The model under review builds one solid part; all positions refer to its coordinate system, in mm. Face numbers are marked on the shaded views. A direction names the side the tool comes from. Coordinates: 2 decimals unless noted, no trailing zeros. Order: outer loops, then holes, each group sorted by start corner. A loop starts at its lowest first (then second) coordinate and runs counter-clockwise, first axis right, second up.
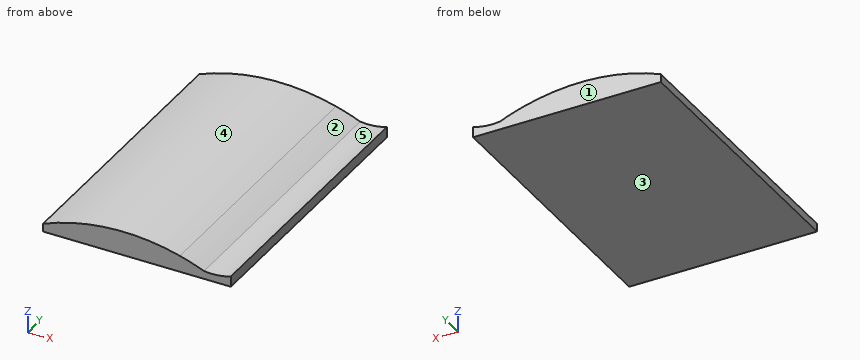
```python
from build123d import *

# Parameters (mm, degrees)
F1_DEPTH = 266.7
F2_DEPTH = 266.7


with BuildPart() as f1:
    # F0 (on Front) → F1 (new body)
    with BuildSketch(Plane.XZ):
        with BuildLine():
            Line((1.9e-05, 0), (1.9e-05, 15.544557))
            ThreePointArc((1.9e-05, 15.544557), (-65.437277, 22.490322), (-129.539981, 7.62))
            Line((-129.539981, 7.62), (-129.539981, 0))
            Line((-129.539981, 0), (1.9e-05, 0))
        make_face()
    extrude(amount=F1_DEPTH)

    # F0 (on Front) → F2 (join)
    with BuildSketch(Plane.XZ):
        with BuildLine():
            Line((1.9e-05, 0), (1.9e-05, 15.544557))
            ThreePointArc((1.9e-05, 15.544557), (-65.437277, 22.490322), (-129.539981, 7.62))
            Line((-129.539981, 7.62), (-129.539981, 0))
            Line((-129.539981, 0), (1.9e-05, 0))
        make_face()
        with BuildLine():
            ThreePointArc((48.260019, 10.16), (35.713201, 7.358175), (22.860019, 7.62))
            ThreePointArc((22.860019, 7.62), (11.551101, 11.931565), (1.9e-05, 15.544557))
            Line((1.9e-05, 15.544557), (1.9e-05, 0))
            Line((1.9e-05, 0), (48.260019, 0))
            Line((48.260019, 0), (48.260019, 10.16))
        make_face()
    extrude(amount=F2_DEPTH)


solid = f1.part
```
(1) We need section A-A, the plane y = -60. Write out the cut boundary in (x, z), and give its area (3 significant figures).
A:
outline: (-129.54, 0) - (48.26, 0) - (48.26, 10.16) arc R53.68 cw to (22.86, 7.62) arc R198.12 ccw to (0, 15.54) arc R198.12 ccw to (-129.54, 7.62) - close
area: 2,920 mm2
(2) We need section C-C, the plane x = -104. Write out the cut boundary in (y, z).
A:
outline: (-266.7, 0) - (0, 0) - (0, 16.27) - (-266.7, 16.27) - close
(3) We need section B-B, the plane x = 36.5. Write out the cut boundary in (y, z), and give its area (3 significant figures).
A:
outline: (-266.7, 0) - (0, 0) - (0, 7.44) - (-266.7, 7.44) - close
area: 1,980 mm2
(4) For pin 1 Ø12 at (x, y) = (-83.5, -137.5) entering from +Z, flat-tipped, find the tip position at first contact; note if it passes through.
A:
pin 1: stops at z = 21.38
(5) Machinability: for the marked faces 1 and 2, which of the approach directions +Z, -Z, +X, -X, +Y, -Y give a long, thin tool a straight path to every point of the face, cutting with its end or side? Answer none if there is none.
A:
face 1: +Z, -Z, +X, -X, +Y
face 2: +Z, +Y, -Y
(6) Draft analysis for pull direction X (two halves, no side actions). For the marked faces 3, 4 and 5, state which applies: released by +X, released by -X, zero draft, split by the parting line, or undercut.
A:
face 3: zero draft
face 4: split by the parting line
face 5: undercut
(7) Wall thickness on probe 1 along Z at (x, y) = (-20.5, -62.5); probe 2 along Z at (x, y) = (-40, -196.5): over which ranges is each line inside the solid? List them lowest first.
A:
probe 1: z = 0 to 20.12
probe 2: z = 0 to 22.41
